Design review of the part built by this model. Coordinates are the model's own, in mm. Face numbers are marked on the shaded views. A direction names the side the tool comes from. Round coordinates to 2 decimals unless told otherwise and drop trailing zeros. Order: outer loops, then holes, each group sorted by start corner. A loop starts at its lowest first (then second) coordinate and runs counter-clockwise, first axis right, second up.
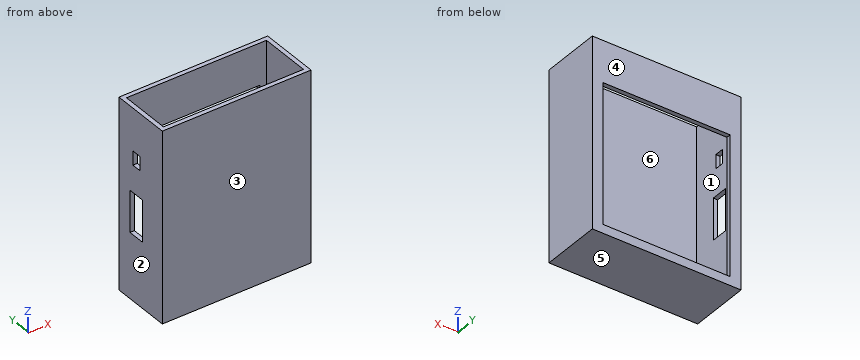
from build123d import *

# Parameters (mm, degrees)
SKETCH_1_W            = 32
SKETCH_1_H            = 42.4
EXTRUDE_1_DEPTH       = 11.7
SHELL_1_T             = 1
CUT_EXTRUDE_664_REACH = 58.36
SKETCH_2_W            = 9.5
SKETCH_2_H            = 3.9
SKETCH_4_W            = 34
SKETCH_4_H            = 43.4
SKETCH_4_W_2          = 29
SKETCH_4_H_2          = 31.9
EXTRUDE_2_DEPTH       = 1


with BuildPart() as part:
    # 草图1 → 凸台-拉伸1 (new body)
    with BuildSketch(Plane(origin=(0, 0, 0), x_dir=(1, 0, 0), z_dir=(0, 1, 0))):
        with Locations((16, 21.2)):
            Rectangle(SKETCH_1_W, SKETCH_1_H)
    extrude(amount=EXTRUDE_1_DEPTH)

    # 抽壳1
    shell_1_openings = [part.faces().sort_by_distance(p)[0] for p in [
        (16, 5.85, 0),
        (16, 11.7, -21.2),
    ]]
    offset(amount=SHELL_1_T, openings=shell_1_openings, kind=Kind.INTERSECTION)

    # 草图2 → Cut-Extrude 664 (cut, up to next)
    with BuildSketch(Plane.ZY.offset(1), mode=Mode.PRIVATE) as cut_extrude_664_sk1:
        with Locations((-23.75, 7.25)):
            Rectangle(SKETCH_2_W, SKETCH_2_H)
    cut_extrude_664_tool1 = extrude(cut_extrude_664_sk1.sketch, amount=-CUT_EXTRUDE_664_REACH, mode=Mode.PRIVATE) & part.part
    # 草图2 → Cut-Extrude 664 (cut, up to next)
    with BuildSketch(Plane.ZY.offset(1), mode=Mode.PRIVATE) as cut_extrude_664_sk2:
        Polygon((-11.25, 8.3), (-9.65, 8.3), (-9.65, 6.1), (-12.85, 6.1), (-12.85, 8.3), align=None)
    cut_extrude_664_tool2 = extrude(cut_extrude_664_sk2.sketch, amount=-CUT_EXTRUDE_664_REACH, mode=Mode.PRIVATE) & part.part
    add(cut_extrude_664_tool1.solids().sort_by_distance((-1, 7.25, -23.75))[0], mode=Mode.SUBTRACT)
    add(cut_extrude_664_tool2.solids().sort_by_distance((-1, 7.2, -11.25))[0], mode=Mode.SUBTRACT)

    # 草图4 → 凸台-拉伸2 (add)
    with BuildSketch(Plane(origin=(0, 11.7, 0), x_dir=(1, 0, 0), z_dir=(0, 1, 0))):
        with Locations((16, 21.7)):
            Rectangle(SKETCH_4_W, SKETCH_4_H)
        with Locations((16, 25.45)):
            Rectangle(SKETCH_4_W_2, SKETCH_4_H_2, mode=Mode.SUBTRACT)
    extrude(amount=EXTRUDE_2_DEPTH)


solid = part.part
1) The part is to be moulded in two halves that separate along Y. For the marked faces 1, 2, 3 and 4, say which applies: released by +Y, released by -Y, zero draft, split by the parting line, or undercut.
Results:
face 1: undercut
face 2: zero draft
face 3: released by -Y
face 4: released by +Y
2) To check wall thickness, follow line 1 along Y through (x, z) = (31.5, -1.5); line 2 along X through (y, z) = (4.75, -10.5); line 3 along X through (y, z) = (11.75, -34). State the ranges of each line that lie inside material, in increasing order.
Results:
line 1: y = -1 to 0, 11.7 to 12.7
line 2: x = -1 to 0, 32 to 33
line 3: x = -1 to 1.5, 30.5 to 33
3) Take a section at D-D on z = -26.5. Give the boundary of the cut face in (x, y).
Results:
outline: (-1, -1) - (33, -1) - (33, 12.7) - (30.5, 12.7) - (30.5, 11.7) - (32, 11.7) - (32, 0) - (0, 0) - (0, 5.3) - (-1, 5.3) - close; (-1, 9.2) - (0, 9.2) - (0, 11.7) - (1.5, 11.7) - (1.5, 12.7) - (-1, 12.7) - close
4) For the marked faces 5 and 6, list the 3-axis set-ups (+Z, -Z, +X, -X, +Y, -Y) from which the entire face can be reached by the end or side of a thin tool; tool diameter is ignored.
Results:
face 5: -Z, +X, -X, +Y, -Y
face 6: +Z
5) Take a section at A-A on z = -10.5. Give the boundary of the cut face in (x, y), plus the area to 3 significant figures.
Results:
outline: (-1, -1) - (33, -1) - (33, 12.7) - (30.5, 12.7) - (30.5, 11.7) - (32, 11.7) - (32, 0) - (0, 0) - (0, 6.1) - (-1, 6.1) - close; (-1, 8.3) - (0, 8.3) - (0, 11.7) - (1.5, 11.7) - (1.5, 12.7) - (-1, 12.7) - close
area: 60.2 mm2
6) Take a section at B-B on x = 17. Give the boundary of the cut face in (y, z).
Results:
outline: (-1, -43.4) - (12.7, -43.4) - (12.7, -41.4) - (11.7, -41.4) - (11.7, -42.4) - (0, -42.4) - (0, 0) - (-1, 0) - close; (11.7, -9.5) - (12.7, -9.5) - (12.7, 0) - (11.7, 0) - close
7) Clearance check with a flat-ended pin moving along its axis: P1, Ø3, axis at x = 12.5, y = 8.5, coming from the +Z side. State where the tip first meets the part, or that it passes through.
Results:
P1: stops at z = -42.4
8) Take a section at C-C on y = 2.5. Give the boundary of the cut face in (x, z), plus the area to 3 significant figures.
Results:
outline: (-1, -43.4) - (33, -43.4) - (33, 0) - (32, 0) - (32, -42.4) - (0, -42.4) - (0, 0) - (-1, 0) - close
area: 119 mm2
